Autodesk Inventor part; units mm, degrees
ref_plane "housing_to_dummy_XY" through (0, 0, 0) normal (0, 0, 1) x (1, 0, 0)
ref_plane "housing_to_dummy_YZ" through (0, 0, 0) normal (1, 0, 0) x (0, 1, 0)
ref_plane "housing_to_dummy_ZX" through (0, 0, 0) normal (0, 1, 0) x (0, 0, 1)
sketch "Sketch_1" plane through (0, 0, 0) normal (1, 0, 0) x (0, 0, -1)
  line L0 (-13, 15.1987) -> (-13, -15.1987)
  arc A0 (-13, -15.1987) -> (13, -15.1987) centre (0, 0) ccw
  line L1 (13, -15.1987) -> (13, 15.1987)
  arc A1 (13, 15.1987) -> (-13, 15.1987) centre (0, 0) ccw
extrude "Extrusion1" add sketch "Sketch_1" along normal mid plane 8
sketch "Sketch2" plane through (-4, 0, 0) normal (-1, 0, 0) x (0, 0, 1)
  point P0 (0, 0)
hole "Hole1" at (-4, 0, 0) direction (1, 0, 0) diameter 19 depth 8 counterbore diameter 22 counterbore depth 6
sketch "Sketch_11" plane through (0, 0, 0) normal (0, 0, 1) x (1, 0, 0)
  line L0 (4, -15.5) -> (-4, -15.5)
  line L1 (-4, -15.5) -> (-4, -13)
  line L2 (-4, -13) -> (-3.567, -13.433)
  line L3 (-3.567, -13.433) -> (3.567, -13.433)
  line L4 (3.567, -13.433) -> (4, -13)
  line L5 (4, -13) -> (4, -15.5)
  line L6 (4, -15.5) -> (-4, -15.5)
revolve "Revolution1" cut sketch "Sketch_11" angle 360 about axis through (4, -15.5, 0) along (1, 0, 0)
thread "Thread1"
sketch "Sketch_9" plane through (0, 0, 0) normal (0, 0, 1) x (1, 0, 0)
  line L0 (4, 15.5) -> (-4, 15.5)
  line L1 (-4, 15.5) -> (-4, 18)
  line L2 (-4, 18) -> (-3.567, 17.567)
  line L3 (-3.567, 17.567) -> (3.567, 17.567)
  line L4 (3.567, 17.567) -> (4, 18)
  line L5 (4, 18) -> (4, 15.5)
  line L6 (4, 15.5) -> (-4, 15.5)
revolve "Revolution2" cut sketch "Sketch_9" angle 360 about axis through (4, 15.5, 0) along (1, 0, 0)
thread "Thread2"
ref_plane "housing_to_dummy_XY" through (0, 0, 0) normal (0, 0, 1) x (1, 0, 0)
ref_plane "housing_to_dummy_YZ" through (0, 0, 0) normal (1, 0, 0) x (0, 1, 0)
ref_plane "housing_to_dummy_ZX" through (0, 0, 0) normal (0, 1, 0) x (0, 0, 1)
ref_plane "to_bearings_XY" through (-4, 0, 0) normal (-1, 0, 0) x (0, 0, -1)
ref_plane "to_bearings_YZ" through (-4, 0, 0) normal (0, 0, -1) x (0, -1, 0)
ref_plane "to_bearings_ZX" through (-4, 0, 0) normal (0, -1, 0) x (-1, 0, 0)
properties part number "SBGTN6900VV_h"
Read the model definition and answer for the solid it produces. Units are mm, in the model's axes. A direction names the side the tool comes from. Give positions to 0.01 mm unless a question says otherwise; leave off trailing zeros. Order: outer loops, then holes, each group sorted by start corner. A loop starts at its lowest first (then second) coordinate and runs counter-clockwise, first axis right, second up.
(1) For faces 1 (the cylindrical face through (3.01, 8.43, 4.38)), 2 (the cylindrical face through (-0.96, 10.74, -2.38)), determine the directions among +Z, -Z, +X, -X, +Y, -Y from which every point of the face is accessible in a straight line to the end or side of a thin tool.
(2) Straight lines are drawn through the part: L1, parallel to Z at x = -1.9, y = 0; L2, parallel to Z at x = 2.8, y = 0; L3, parallel to Y at x = -2, z = -0.75. For each, find the intervals that lie inside material, in ascending order.
(3) Find section A-A (z = 5.25). Give the vertices of the cut face in (x, y).
(4) For a pull along Y with two mould halves and no side action, classify faces 3 (the flat face through (0, 0, 13)), 4 (the cylindrical face through (0.05, 17.47, 0.62)), 5 (the cylindrical face through (0, -20, 0)) as released by +Y, released by -Y, zero draft, split by the parting line, or undercut.
(5) Find section C-C (z = 0). Give the vertices of the cut face in (x, y).
(6) Given pin 1 (3.5 mm diameter, centred on y = -15.5, z = 0, fed in from +X), flat-ended and moving along its own axis, determine where the tip first touches the part or whether it passes through.
(7) Find section D-D (x = -2.25). Give the vertices of the cut face in (y, z).
(8) Find section B-B (y = 0). Give the vertices of the cut face in (x, z), plus the area to 3 significant figures.
Result sheet:
1. face 1: +X, -X
1. face 2: -X
2. L1: z = -13 to -11, 11 to 13
2. L2: z = -13 to -9.5, 9.5 to 13
2. L3: y = -19.99 to -17.43, -13.57 to -10.97, 10.97 to 13.57, 17.43 to 19.99
3. outline: (-4, -19.3) - (4, -19.3) - (4, -7.92) - (2, -7.92) - (2, -9.67) - (-4, -9.67) - close; (-4, 9.67) - (2, 9.67) - (2, 7.92) - (4, 7.92) - (4, 19.3) - (-4, 19.3) - close
4. face 3: zero draft
4. face 4: undercut
4. face 5: released by -Y
5. outline: (-4, -20) - (4, -20) - (4, -18) - (3.57, -17.57) - (-3.57, -17.57) - (-4, -18) - close; (-4, -13) - (-3.57, -13.43) - (3.57, -13.43) - (4, -13) - (4, -9.5) - (2, -9.5) - (2, -11) - (-4, -11) - close; (-4, 11) - (2, 11) - (2, 9.5) - (4, 9.5) - (4, 13) - (3.57, 13.43) - (-3.57, 13.43) - (-4, 13) - close; (-4, 18) - (-3.57, 17.57) - (3.57, 17.57) - (4, 18) - (4, 20) - (-4, 20) - close
6. pin 1: passes through
7. outline: (-15.2, -13) - (15.2, -13) arc R20 ccw to (15.2, 13) - (-15.2, 13) arc R20 ccw to start; hole circle Ø4.13 at (-15.5, 0); hole circle Ø22 at (0, 0); hole circle Ø4.13 at (15.5, 0)
8. outline: (-4, -13) - (4, -13) - (4, -9.5) - (2, -9.5) - (2, -11) - (-4, -11) - close; (-4, 11) - (2, 11) - (2, 9.5) - (4, 9.5) - (4, 13) - (-4, 13) - close
8. area: 38.0 mm2
